The model under review builds one solid part; all positions refer to its coordinate system, in mm. Round coordinates to 2 decimals unless told otherwise and drop trailing zeros. One line per question, with ' | ' between items.
from build123d import *

# Parameters (mm, degrees)
F0_W     = 166
F0_H     = 96
F0_R     = 1
F1_DEPTH = 2
F3_D     = 5
F3_DEPTH = 12
F3_TIP   = 1.5021515476
F4_D     = 2.75
F4_DEPTH = 12
F4_TIP   = 0.8261833512
F5_D     = 7
F5_DEPTH = 12
F5_TIP   = 2.1030121666


with BuildPart() as f1:
    # F0 (on Top) → F1 (new body)
    with BuildSketch(Plane.XY):
        with Locations((15.2820143104, 21.6586496021)):
            Rectangle(F0_W, F0_H)
        with Locations((-64.7179856896, -23.3413503979)):
            Circle(F0_R, mode=Mode.SUBTRACT)
        with Locations((95.2820143104, -23.3413503979)):
            Circle(F0_R, mode=Mode.SUBTRACT)
        with Locations((-64.7179856896, 66.6586496021)):
            Circle(F0_R, mode=Mode.SUBTRACT)
        with Locations((95.2820143104, 66.6586496021)):
            Circle(F0_R, mode=Mode.SUBTRACT)
    extrude(amount=F1_DEPTH)

    # F3
    with Locations(Plane(origin=(0, 0, 0), x_dir=(1, 0, 0), z_dir=(0, 0, -1))):
        with Locations((83.2820143104, -59.6586496021), (83.2820143104, -7.9086496021)):
            Hole(F3_D / 2, depth=F3_DEPTH)
            with Locations((0, 0, -(F3_DEPTH + F3_TIP / 2))):  # 118° drill point
                Cone(0, F3_D / 2, F3_TIP, mode=Mode.SUBTRACT)

    # F4
    with Locations(Plane(origin=(0, 0, 0), x_dir=(1, 0, 0), z_dir=(0, 0, -1))):
        with Locations((-29.2179856896, -61.1586496021), (-29.2179856896, -12.1586496021), (28.7820143104, -12.1586496021), (28.7820143104, -61.1586496021)):
            Hole(F4_D / 2, depth=F4_DEPTH)
            with Locations((0, 0, -(F4_DEPTH + F4_TIP / 2))):  # 118° drill point
                Cone(0, F4_D / 2, F4_TIP, mode=Mode.SUBTRACT)

    # F5
    with Locations(Plane(origin=(0, 0, 0), x_dir=(1, 0, 0), z_dir=(0, 0, -1))):
        with Locations((-56.0955218971, 7.4801053852), (86.1625224352, 7.4801053852), (42.0048907399, -12.1859554201)):
            Hole(F5_D / 2, depth=F5_DEPTH)
            with Locations((0, 0, -(F5_DEPTH + F5_TIP / 2))):  # 118° drill point
                Cone(0, F5_D / 2, F5_TIP, mode=Mode.SUBTRACT)


solid = f1.part
1) Insertion check: P1, Ø3.5, axis at x = -29.22, y = 12.16, coming from the -Z side. The pin has a flat end and moves straight along its axis. Give the tip position at first contact, or say it passes through.
Output values:
P1: stops at z = 0
2) Mouldability with a two-part tool opening along Y and no side actions: class faces 1 (the flat face through (14, 22, 2)), 2 (the cylindrical face through (85.266, 61.18, 1.014)) as +Y half, -Y half, draft (parallel to the pull), parting line (faces both ways), or undercut.
Output values:
face 1: draft | face 2: undercut
3) For line 1 (X direction, y = -7, z = 1.75); line 2 (Y direction, x = -57.5, z = 1.6); line 3 (Y direction, x = 45, z = 1.8), list the stretches that pass through material, from the lowest coordinate up.
Output values:
line 1: x = -67.72 to -59.56, -52.63 to 82.7, 89.63 to 98.28 | line 2: y = -26.34 to -10.69, -4.27 to 69.66 | line 3: y = -26.34 to 10.38, 14 to 69.66
